Can you work these out from the model? Positions are in its coordinate system, mm. Face numbers are marked on the shaded views. A direction names the side the tool comes from. Coordinates: 2 decimals unless noted, no trailing zeros. Order: outer loops, then holes, each group sorted by start corner. A loop starts at its lowest first (then second) coordinate and runs counter-clockwise, first axis right, second up. Notation, with made-up numbers: (57.25, 56.5) -> (99.25, 56.5) arc R15 cw to (99.25, 75.5) -> close; hole circle Ø3 at (72.5, 34.25). An arc over 180 degrees is marked (long way). Write item = value, one per line.
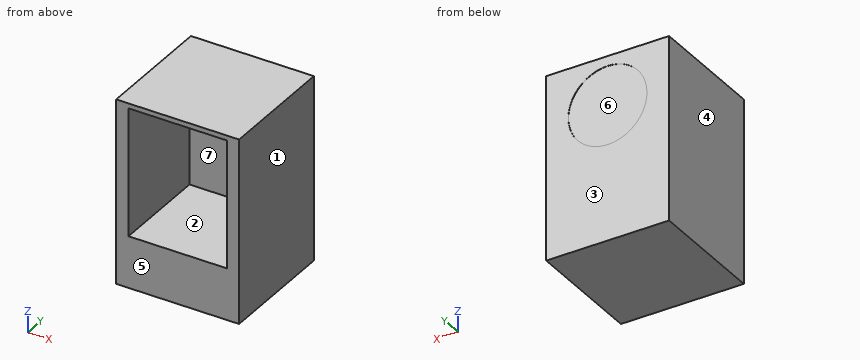
```python
from build123d import *

# Parameters (mm, degrees)
SKETCH1_W           = 75
SKETCH1_H           = 49
BOSS_EXTRUDE1_DEPTH = 50
SKETCH2_W           = 40
SKETCH2_H           = 52
CUT_EXTRUDE1_DEPTH  = 40
SKETCH3_R           = 16
CUT_EXTRUDE3_DEPTH  = 0.1


with BuildPart() as part:
    # Sketch1 → Boss-Extrude1 (new body)
    with BuildSketch(Plane(origin=(0, 0, 0), x_dir=(0, 0, -1), z_dir=(1, 0, 0))):
        Rectangle(SKETCH1_W, SKETCH1_H)
    extrude(amount=BOSS_EXTRUDE1_DEPTH)

    # Sketch2 → Cut-Extrude1 (cut)
    with BuildSketch(Plane.XZ.offset(24.5)):
        with Locations((25, 9.5)):
            Rectangle(SKETCH2_W, SKETCH2_H)
    extrude(amount=-CUT_EXTRUDE1_DEPTH, mode=Mode.SUBTRACT)

    # Sketch3 → Cut-Extrude3 (cut)
    with BuildSketch(Plane(origin=(0, 24.5, 0), x_dir=(1, 0, 0), z_dir=(0, 1, 0))):
        with Locations(Location((25, -17.5, 0), (0, 0, 270))):
            Circle(SKETCH3_R)
    extrude(amount=-CUT_EXTRUDE3_DEPTH, mode=Mode.SUBTRACT)


solid = part.part
```
Item 1: I want a section at D-D, the plane x = 25. Please give me the cut outline in (y, z).
A:
outline = (-24.5, -37.5) -> (24.5, -37.5) -> (24.5, 1.5) -> (24.4, 1.5) -> (24.4, 33.5) -> (24.5, 33.5) -> (24.5, 37.5) -> (-24.5, 37.5) -> (-24.5, 35.5) -> (15.5, 35.5) -> (15.5, -16.5) -> (-24.5, -16.5) -> close
Item 2: If I drill on probe 1 along X at (y, z) = (13.5, -8.5); probe 2 along X at (y, z) = (24.45, 17.5); probe 3 along Z at (x, y) = (9.5, -17), over which ranges is the centre line in solid material (lowest first)?
A:
probe_1 = 0 to 5, 45 to 50
probe_2 = 0 to 9, 41 to 50
probe_3 = -37.5 to -16.5, 35.5 to 37.5
Item 3: I want a section at B-B, the plane z = -11. Please give me the cut outline in (x, y).
A:
outline = (0, -24.5) -> (5, -24.5) -> (5, 15.5) -> (45, 15.5) -> (45, -24.5) -> (50, -24.5) -> (50, 24.5) -> (0, 24.5) -> close
Item 4: I want a section at C-C, the plane y = 0. Please give me the cut outline in (x, z).
A:
outline = (0, -37.5) -> (50, -37.5) -> (50, 37.5) -> (0, 37.5) -> close; hole (5, -16.5) -> (45, -16.5) -> (45, 35.5) -> (5, 35.5) -> close
Item 5: I'm going to push flat-ended pins straight in: P1, Ø20, axis at x = 32, z = 12, coming from the -Y side; P2, Ø12, axis at x = 20.5, z = 23, coming from the +Y side. Where does each tip first touch, or does it pass through?
A:
P1 = 15.5
P2 = 24.4
Item 6: For the marked faces 5, 6 and 7, which set-ups out of +Z, -Z, +X, -X, +Y, -Y let a thin tool reach every point of the face, with its end or its side?
A:
face_5 = +Z, -Z, +X, -X, -Y
face_6 = +Y
face_7 = -Y
Item 7: I want a section at A-A, the plane x = 7. Please give me the cut outline in (y, z), plus the area to 4 significant figures.
A:
outline = (-24.5, -37.5) -> (24.5, -37.5) -> (24.5, 37.5) -> (-24.5, 37.5) -> (-24.5, 35.5) -> (15.5, 35.5) -> (15.5, -16.5) -> (-24.5, -16.5) -> close
area = 1,595 mm2
Item 8: If we mould it in two halves opening along X, with no side actions, what happens to the marked faces 1, 2, 3 and 4? For each: pulls with the +X half, pulls with the -X half, needs draft (parallel to the pull), parting line crosses it, or undercut.
A:
face_1 = pulls with the +X half
face_2 = undercut
face_3 = needs draft
face_4 = pulls with the -X half
